Work out the finished part from the listing and answer in its coordinate system (mm). Round coordinates to 2 decimals unless told otherwise and drop trailing zeros.
```python
from build123d import *

# Parameters (mm, degrees)
SKETCH_1_W          = 9
SKETCH_1_H          = 6.5
EXTRUDE_1_DEPTH     = 250
SKETCH_2_R          = 1.5
CUT_EXTRUDE_1_DEPTH = 250


with BuildPart() as part:
    # 草图1 → 凸台-拉伸1 (new body)
    with BuildSketch(Plane.XY):
        Rectangle(SKETCH_1_W, SKETCH_1_H)
    extrude(amount=EXTRUDE_1_DEPTH)

    # 草图2 → 切除-拉伸1 (cut)
    with BuildSketch(Plane(origin=(0, 3.25, 0), x_dir=(1, 0, 0), z_dir=(0, 1, 0))):
        with Locations(Location((0, -4, 0), (0, 0, 270))):
            Circle(SKETCH_2_R)
        with Locations(Location((0, -24, 0), (0, 0, 270))):
            Circle(SKETCH_2_R)
        with Locations(Location((0, -44, 0), (0, 0, 270))):
            Circle(SKETCH_2_R)
        with Locations(Location((0, -64, 0), (0, 0, 270))):
            Circle(SKETCH_2_R)
        with Locations(Location((0, -84, 0), (0, 0, 270))):
            Circle(SKETCH_2_R)
        with Locations(Location((0, -104, 0), (0, 0, 270))):
            Circle(SKETCH_2_R)
        with Locations(Location((0, -124, 0), (0, 0, 270))):
            Circle(SKETCH_2_R)
        with Locations(Location((0, -144, 0), (0, 0, 270))):
            Circle(SKETCH_2_R)
        with Locations(Location((0, -164, 0), (0, 0, 270))):
            Circle(SKETCH_2_R)
        with Locations(Location((0, -184, 0), (0, 0, 270))):
            Circle(SKETCH_2_R)
        with Locations(Location((0, -204, 0), (0, 0, 270))):
            Circle(SKETCH_2_R)
        with Locations(Location((0, -224, 0), (0, 0, 270))):
            Circle(SKETCH_2_R)
        with Locations(Location((0, -244, 0), (0, 0, 270))):
            Circle(SKETCH_2_R)
    extrude(amount=-CUT_EXTRUDE_1_DEPTH, mode=Mode.SUBTRACT)


solid = part.part
```
1. Given pin 1 (2.5 mm diameter, centred on x = 0, z = 44, fed in from +Y), flat-ended and moving along its own axis, determine where the tip first touches the part or whether it passes through.
Answer key:
pin 1: passes through
2. Find section A-A (y = 1.5). Give the number of separate pieces and of enclosed holes in the cut face, then the cut area to 3 significant figures.
Answer key:
separate pieces: 1
enclosed holes: 13
area: 2,160 mm2
3. Consider probe 1 along X at (y, z) = (1.5, 204). Determine where the line is inside the solid, lowest interval first.
Answer key:
probe 1: x = -4.5 to -1.5, 1.5 to 4.5
